Drawing for the job (mm, zero at the part's lowest x, y, z). A direction names the side the tool comes from. Coordinates: 2 decimals unless noted, no trailing zeros. Write each loop counter-clockwise with the first axis right and the second up, starting at its lowest first coordinate (ties: lowest second). Pieces come first, ordered by that corner, then holes. Notation, with made-up numbers: M 9,-16.75 L 15,-16.75 A8 ccw 15,-12.75 Z; hole C 40.25,78.5 d9. An arc over 180 degrees is marked long. Use a Markdown table: item, result. Add a question column.
Q1. Mould opens along X. For the marked faces 1, 2, 3 and 4 say: released by +X, released by -X, zero draft, split by the parting line, or undercut.
Q2. Slice it at B-B on x = 19.5. Write the cut outline in (y, z), then the cut area to 3 significant figures.
Q3. Wall check: L1, parallel to X at y = 11, z = 21.5; L2, parallel to Z at x = 31.5, y = 8.5; L3, parallel to Z at x = 67, y = 3.5. Give the ranges that are in metal, low to high. Write a range as from..to.
Q4. Slice it at A-A on z = 65.5. Write the cut outline in (x, y), then the cut area to 3 significant figures.
Q5. Tool access for the marked faces 5 and 6: list every direction of +Z, -Z, +X, -X, +Y, -Y with a clear straight run to the whole face (end or side of a thin tool).
Q6. Pin check, flat tips, straight feed: pin 1 Ø1 at (x, z) = (46, 67.5) entering from -Y; pin 2 Ø20 at (x, z) = (97.5, 59.5) entering from +Y. Stop position of each tip, or through.
Q7. Slice it at C-C on y = 10.5. Count the separate pieces of the cut face and the enclosed holes in it.
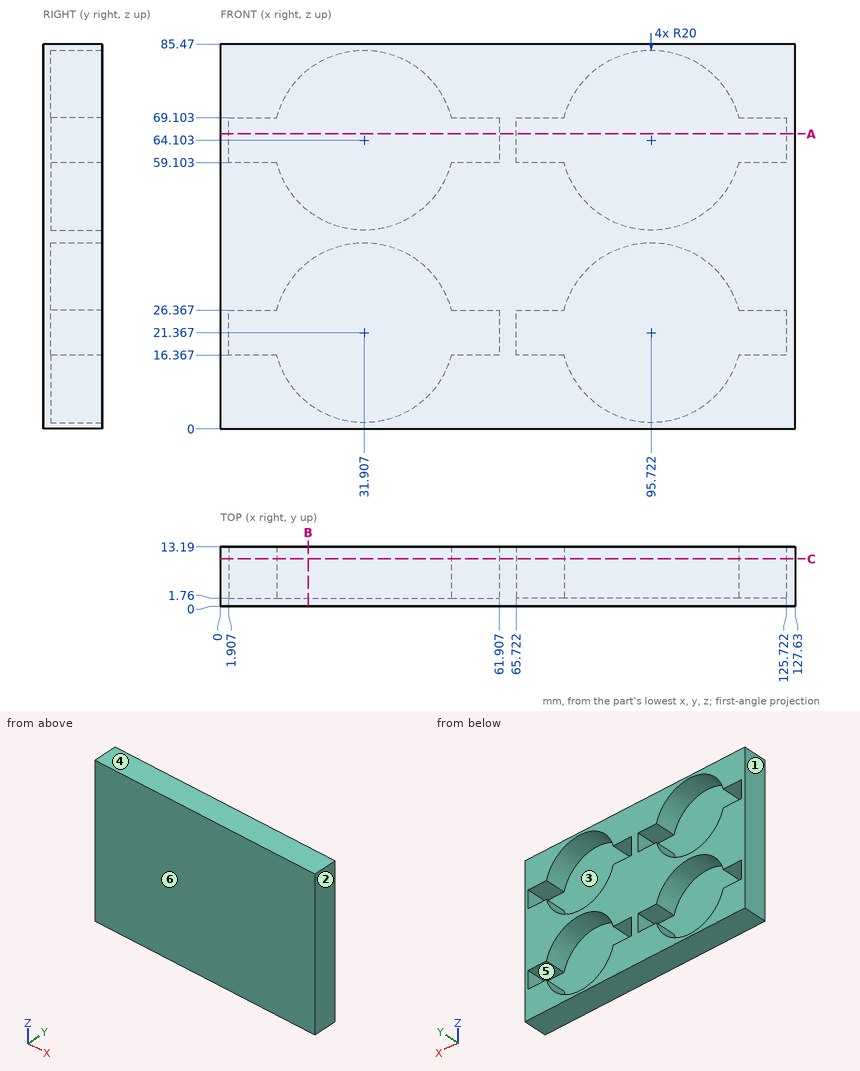
Recorded:
| question | item | result |
|---|---|---|
| 1 | face 1 | released by -X |
| 1 | face 2 | released by +X |
| 1 | face 3 | undercut |
| 1 | face 4 | zero draft |
| 2 | outline | M 0,0 L 13.19,0 L 13.19,5.68 L 1.76,5.68 L 1.76,37.05 L 13.19,37.05 L 13.19,48.42 L 1.76,48.42 L 1.76,79.79 L 13.19,79.79 L 13.19,85.47 L 0,85.47 Z |
| 2 | area | 410 mm² |
| 3 | L1 | 0..1.91, 61.91..65.72, 125.72..127.63 |
| 3 | L2 | 0..1.37, 41.36..44.11, 84.1..85.47 |
| 3 | L3 | 0..16.37, 26.37..59.1, 69.1..85.47 |
| 4 | outline | M 0,0 L 127.63,0 L 127.63,13.19 L 125.72,13.19 L 125.72,1.76 L 65.72,1.76 L 65.72,13.19 L 61.91,13.19 L 61.91,1.76 L 1.91,1.76 L 1.91,13.19 L 0,13.19 Z |
| 4 | area | 312 mm² |
| 5 | face 5 | +Y |
| 5 | face 6 | +Z, -Z, +X, -X, -Y |
| 6 | pin 1 | y = 0 |
| 6 | pin 2 | y = 1.76 |
| 7 | separate pieces | 1 |
| 7 | enclosed holes | 4 |
